from build123d import *

# Parameters (mm, degrees)
SKETCH1_R           = 1.65
SKETCH1_R_2         = 5
BOSS_EXTRUDE1_DEPTH = 3
CUT_EXTRUDE1_DEPTH  = 3
FILLET1_R           = 0.5


with BuildPart() as part:
    # Sketch1 → Boss-Extrude1 (new body)
    with BuildSketch(Plane(origin=(0, 0, 0), x_dir=(0, 0, -1), z_dir=(1, 0, 0))):
        Polygon((-125, 13.75), (-125, -13.75), (-108.645833333, -13.75), (-108.645833333, -10.75), (-92.291666667, -10.75), (-92.291666667, -13.75), (-75.9375, -13.75), (-75.9375, -10.75), (-59.583333333, -10.75), (-59.583333333, -13.75), (-43.229166667, -13.75), (-43.229166667, -10.75), (-26.875, -10.75), (-26.875, -13.75), (-10.520833333, -13.75), (-10.520833333, -10.75), (5.833333333, -10.75), (5.833333333, -13.75), (22.1875, -13.75), (22.1875, -10.75), (38.541666667, -10.75), (38.541666667, -13.75), (125, -13.75), (125, 13.75), (38.541666667, 13.75), (38.541666667, 10.75), (22.1875, 10.75), (22.1875, 13.75), (5.833333333, 13.75), (5.833333333, 10.75), (-10.520833333, 10.75), (-10.520833333, 13.75), (-26.875, 13.75), (-26.875, 10.75), (-43.229166667, 10.75), (-43.229166667, 13.75), (-59.583333333, 13.75), (-59.583333333, 10.75), (-75.9375, 10.75), (-75.9375, 13.75), (-92.291666667, 13.75), (-92.291666667, 10.75), (-108.645833333, 10.75), (-108.645833333, 13.75), align=None)
        with Locations((103.25, -8)):
            Circle(SKETCH1_R, mode=Mode.SUBTRACT)
        with Locations((119.25, -8)):
            Circle(SKETCH1_R, mode=Mode.SUBTRACT)
        with Locations((-111.25, 0)):
            Circle(SKETCH1_R_2, mode=Mode.SUBTRACT)
        with BuildLine():
            Line((95.5778, -6.2), (75.1778, -6.2))
            ThreePointArc((75.1778, -6.2), (74.648857766, 0), (75.1778, 6.2))
            Line((75.1778, 6.2), (95.5778, 6.2))
            Line((95.5778, 6.2), (95.5778, -6.2))
        make_face(mode=Mode.SUBTRACT)
        with Locations((111.25, 0)):
            Circle(SKETCH1_R_2, mode=Mode.SUBTRACT)
        with Locations((103.25, 8)):
            Circle(SKETCH1_R, mode=Mode.SUBTRACT)
        with Locations((119.25, 8)):
            Circle(SKETCH1_R, mode=Mode.SUBTRACT)
    extrude(amount=BOSS_EXTRUDE1_DEPTH)

    # Sketch3 → Cut-Extrude1 (cut)
    with BuildSketch(Plane(origin=(3, 0, 0), x_dir=(0, 0, -1), z_dir=(1, 0, 0))):
        Polygon((-102.25, 0), (-102.25, -6.25), (-84.139910217, -6.25), align=None)
        Polygon((-55.299825543, 6.25), (-101.661655387, 6.25), (-78.480740465, -1.75), align=None)
        Polygon((-49.640655791, 1.75), (-72.821570713, -6.25), (-26.459740869, -6.25), align=None)
        Polygon((2.380343805, 6.25), (-43.981486039, 6.25), (-20.800571117, -1.75), align=None)
        Polygon((8.039513557, 1.75), (-15.141401365, -6.25), (31.220428479, -6.25), align=None)
        Polygon((60.060513153, 6.25), (13.698683309, 6.25), (36.879598231, -1.75), align=None)
        Polygon((60.648857766, 0), (42.538767983, -6.25), (60.648857766, -6.25), align=None)
    extrude(amount=-CUT_EXTRUDE1_DEPTH, mode=Mode.SUBTRACT)

    # Fillet1
    fillet1_edges = [part.edges().sort_by_distance(p)[0] for p in [
        (1.5, -1.75, 20.800571117),
        (1.5, 6.25, 43.981486039),
        (1.5, 6.25, -2.380343805),
        (1.5, 1.75, -8.039513557),
        (1.5, -6.25, -31.220428479),
        (1.5, -6.25, 15.141401365),
        (1.5, -1.75, 78.480740465),
        (1.5, 6.25, 101.661655387),
        (1.5, 6.25, 55.299825543),
        (1.5, 1.75, 49.640655791),
        (1.5, -6.25, 26.459740869),
        (1.5, -6.25, 72.821570713),
        (1.5, -6.25, -42.538767983),
        (1.5, 0, -60.648857766),
        (1.5, -6.25, -60.648857766),
        (1.5, -1.75, -36.879598231),
        (1.5, 6.25, -13.698683309),
        (1.5, 6.25, -60.060513153),
        (1.5, 0, 102.25),
        (1.5, -6.25, 84.139910217),
        (1.5, -6.25, 102.25),
    ]]
    fillet(fillet1_edges, radius=FILLET1_R)


solid = part.part
Input: part model. Units: mm. Frame: model coordinates. A direction names the side the tool comes from. Give positions to 0.01 mm unless a question says otherwise; leave off trailing zeros. Order: outer loops, then holes, each group sorted by start corner. A loop starts at its lowest first (then second) coordinate and runs counter-clockwise, first axis right, second up.
Q1. Section B-B on x = 1.55. State how many separate pieces and enclosed holes the cut face has, and give its area (3 significant figures).
Checked values:
separate pieces: 1
enclosed holes: 14
area: 4,910 mm2
Q2. Section C-C on z = -53. Output: boundary loops of the cut face in (x, y), and give its area (3 significant figures).
Checked values:
outline: (0, -13.75) - (3, -13.75) - (3, -6.25) - (0, -6.25) - close; (0, -2.64) - (3, -2.64) - (3, 3.81) - (0, 3.81) - close; (0, 6.25) - (3, 6.25) - (3, 13.75) - (0, 13.75) - close
area: 64.4 mm2
Q3. Section A-A on z = -111.25. Output: boundary loops of the cut face in (x, y).
Checked values:
outline: (0, -13.75) - (3, -13.75) - (3, -5) - (0, -5) - close; (0, 5) - (3, 5) - (3, 13.75) - (0, 13.75) - close
Q4. Ray query, probe 1 along Y at (x, z) = (1.45, -103.25); probe 2 along Y at (x, z) = (2.8, -77); probe 3 along Y at (x, z) = (2.35, -111.25). Return the intervals inside material, ascending.
Checked values:
probe 1: y = -13.75 to -9.65, -6.35 to 6.35, 9.65 to 13.75
probe 2: y = -13.75 to -6.2, 6.2 to 13.75
probe 3: y = -13.75 to -5, 5 to 13.75
Q5. Set-up query: faces 3 (the flat face through (3, 0, 2)), 4 (the flat face through (1.52, -2.79, 94.17)). Return all of +Z, -Z, +X, -X, +Y, -Y with unobstructed straight access to the full face (end or side cutting, diameter ignored); none if empty.
Checked values:
face 3: +Z, -Z, +X, +Y, -Y
face 4: +X, -X
Q6. Section D-D on z = 23.5. Output: boundary loops of the cut face in (x, y).
Checked values:
outline: (0, -13.75) - (3, -13.75) - (3, -0.82) - (0, -0.82) - close; (0, 6.25) - (3, 6.25) - (3, 13.75) - (0, 13.75) - close
Q7. Draft query along Y for faces 1 (the flat face through (0, 0, 2)), 2 (the cylindrical face through (1.479, -1.915, 106.631)). Return one class per face: +Y half, -Y half, draft (parallel to the pull), parting line (faces both ways), or undercut.
Checked values:
face 1: draft
face 2: undercut
Q8. Contact query for a flat-ended pin moving along its axis: pin 1 Ø0.9 at (x, z) = (1.5, 104) entering from +Y. Output: stop coordinate, or through.
Checked values:
pin 1: stops at y = 10.75
